from build123d import *

# Parameters (mm, degrees)
F0_R     = 18.7435509256
F1_DEPTH = 25.4


with BuildPart() as f1:
    # F0 (on Front) → F1 (new body)
    with BuildSketch(Plane.XZ):
        with BuildLine():
            Line((-12.5020157932, 38.4971815486), (-6.5838834434, 48.7476874643))
            ThreePointArc((-6.5838834434, 48.7476874643), (-6.5838834434, 71.5549287346), (13.1677668869, 60.1513080994))
            ThreePointArc((13.1677668869, 60.1513080994), (11.4036206351, 53.567424656), (6.5838834434, 48.7476874643))
            Line((6.5838834434, 48.7476874643), (12.5020157932, 38.4971815486))
            ThreePointArc((12.5020157932, 38.4971815486), (21.6541265509, 47.6492923062), (25.0040315864, 60.1513080994))
            ThreePointArc((25.0040315864, 60.1513080994), (-12.5020157932, 81.8054346503), (-12.5020157932, 38.4971815486))
        make_face()
        with BuildLine():
            ThreePointArc((6.5838834434, 48.7476874643), (0, 46.9835412126), (-6.5838834434, 48.7476874643))
            Line((-6.5838834434, 48.7476874643), (-12.5020157932, 38.4971815486))
            ThreePointArc((-12.5020157932, 38.4971815486), (0, 35.147276513), (12.5020157932, 38.4971815486))
            Line((12.5020157932, 38.4971815486), (6.5838834434, 48.7476874643))
        make_face()
        with BuildLine():
            ThreePointArc((12.5020157932, 38.4971815486), (0, 35.147276513), (-12.5020157932, 38.4971815486))
            Line((-12.5020157932, 38.4971815486), (-50.3756712224, -27.1019139232))
            ThreePointArc((-50.3756712224, -27.1019139232), (-40.767995742, -36.7095894036), (-37.2513424448, -49.8339181812))
            Line((-37.2513424448, -49.8339181812), (36.6895705679, -49.8339181812))
            ThreePointArc((36.6895705679, -49.8339181812), (40.2814870254, -36.4287034651), (50.094785284, -26.6154052066))
            Line((50.094785284, -26.6154052066), (12.5020157932, 38.4971815486))
        make_face()
        Circle(F0_R, mode=Mode.SUBTRACT)
        with BuildLine():
            Line((55.796700688, -36.491412387), (50.094785284, -26.6154052066))
            ThreePointArc((50.094785284, -26.6154052066), (40.2814870254, -36.4287034651), (36.6895705679, -49.8339181812))
            Line((36.6895705679, -49.8339181812), (48.0934013761, -49.8339181812))
            ThreePointArc((48.0934013761, -49.8339181812), (50.1574942058, -42.1306188692), (55.796700688, -36.491412387))
        make_face()
        with BuildLine():
            ThreePointArc((90.3104294321, -49.8339181812), (76.905214716, -26.6154052066), (50.094785284, -26.6154052066))
            Line((50.094785284, -26.6154052066), (55.796700688, -36.491412387))
            ThreePointArc((55.796700688, -36.491412387), (71.203299312, -36.491412387), (78.9065986239, -49.8339181812))
            ThreePointArc((78.9065986239, -49.8339181812), (63.5, -65.2405168051), (48.0934013761, -49.8339181812))
            Line((48.0934013761, -49.8339181812), (36.6895705679, -49.8339181812))
            ThreePointArc((36.6895705679, -49.8339181812), (63.5, -76.6443476133), (90.3104294321, -49.8339181812))
        make_face()
        with BuildLine():
            ThreePointArc((-37.2513424448, -49.8339181812), (-40.767995742, -36.7095894036), (-50.3756712224, -27.1019139232))
            Line((-50.3756712224, -27.1019139232), (-55.9869244457, -36.8208896001))
            ThreePointArc((-55.9869244457, -36.8208896001), (-50.4869714189, -42.3208426269), (-48.4738488914, -49.8339181812))
            Line((-48.4738488914, -49.8339181812), (-37.2513424448, -49.8339181812))
        make_face()
        with BuildLine():
            Line((-55.9869244457, -36.8208896001), (-50.3756712224, -27.1019139232))
            ThreePointArc((-50.3756712224, -27.1019139232), (-86.232004258, -62.9582469588), (-37.2513424448, -49.8339181812))
            Line((-37.2513424448, -49.8339181812), (-48.4738488914, -49.8339181812))
            ThreePointArc((-48.4738488914, -49.8339181812), (-76.5130285811, -57.3469937355), (-55.9869244457, -36.8208896001))
        make_face()
    extrude(amount=F1_DEPTH)


solid = f1.part
Source: CAD feature listing. Evaluate the final solid. Frame: model axes, mm. Coordinates: 2 decimals unless noted, no trailing zeros. Write each loop counter-clockwise with the first axis right and the second up, starting at its lowest first coordinate (ties: lowest second). Pieces come first, ordered by that corner, then holes. Notation, with made-up numbers: M -32,-27 L -8,-27 A9 ccw -8,-19 Z; hole C 48,-16.75 d8. An arc over 180 degrees is marked long. Use a Markdown table: item, result.
1) Mould query, pull axis Z, two halves, no side actions, for faces 1 (the flat face through (31.56, -12.52, 5.49)), 2 (the cylindrical face through (-86.698, -12.522, -62.116)), 3 (the flat face through (-1, -13, -49.834)), 4 (the flat face through (-1, -25.4, -31)). Classes: pulls with the +Z half, pulls with the -Z half, needs draft (parallel to the pull), parting line crosses it, or undercut.
Conclusion:
| item | result |
|---|---|
| face 1 | undercut |
| face 2 | parting line crosses it |
| face 3 | pulls with the -Z half |
| face 4 | needs draft |
2) Section A-A, the plane x = 63.5. Output: boundary loops of the cut face in (y, z).
Conclusion:
| item | result |
|---|---|
| outline | M -25.4,-76.64 L 0,-76.64 L 0,-65.24 L -25.4,-65.24 Z; M -25.4,-34.43 L 0,-34.43 L 0,-23.02 L -25.4,-23.02 Z |
3) Section B-B, the plane y = -17. Output: boundary loops of the cut face in (x, z), then the cut area to 3 significant figures.
Conclusion:
| item | result |
|---|---|
| outline | M -50.38,-27.1 A26.25 ccw long -37.25,-49.83 L 36.69,-49.83 A26.81 ccw long 50.09,-26.62 L 12.5,38.5 A25 ccw long -12.5,38.5 Z; hole C -63.5,-49.83 d30.05; hole C 0,0 d37.49; hole C 0,60.15 d26.34; hole C 63.5,-49.83 d30.81 |
| area | 9,200 mm^2 |
4) Ray query, L1, parallel to Z at x = 0, y = -14.5; L2, parallel to X at y = -7.5, z = -41; L3, parallel to Z at x = -63.5, y = -12.25. Return the intervals inside material, ascending.
Conclusion:
| item | result |
|---|---|
| L1 | z = -49.83 to -18.74, 18.74 to 46.98, 73.32 to 85.16 |
| L2 | x = -88.22 to -75.66, -51.34 to 50.88, 76.12 to 88.81 |
| L3 | z = -76.08 to -64.86, -34.81 to -23.59 |
5) Section C-C, the plane x = 0. Output: boundary loops of the cut face in (y, z), then the cut area to 3 significant figures.
Conclusion:
| item | result |
|---|---|
| outline | M -25.4,-49.83 L 0,-49.83 L 0,-18.74 L -25.4,-18.74 Z; M -25.4,18.74 L 0,18.74 L 0,46.98 L -25.4,46.98 Z; M -25.4,73.32 L 0,73.32 L 0,85.16 L -25.4,85.16 Z |
| area | 1,810 mm^2 |
6) Section D-D, the plane z = 5. Output: boundary loops of the cut face in (x, y), then the cut area to 3 significant figures.
Conclusion:
| item | result |
|---|---|
| outline | M -31.84,-25.4 L -18.06,-25.4 L -18.06,0 L -31.84,0 Z; M 18.06,-25.4 L 31.84,-25.4 L 31.84,0 L 18.06,0 Z |
| area | 700 mm^2 |
7) First-contact query: pin 1 Ø8 at (x, y) = (12, -14.5) entering from +Z; pin 2 Ø3 at (x, y) = (15.5, -19) entering from -Z; pin 3 Ø8 at (x, y) = (70.5, -16.5) entering from +Z. Flat tips, straight axial feed; report the tip coordinate or a pass-through.
Conclusion:
| item | result |
|---|---|
| pin 1 | stops at z = 83.84 |
| pin 2 | stops at z = -49.83 |
| pin 3 | stops at z = -23.19 |
